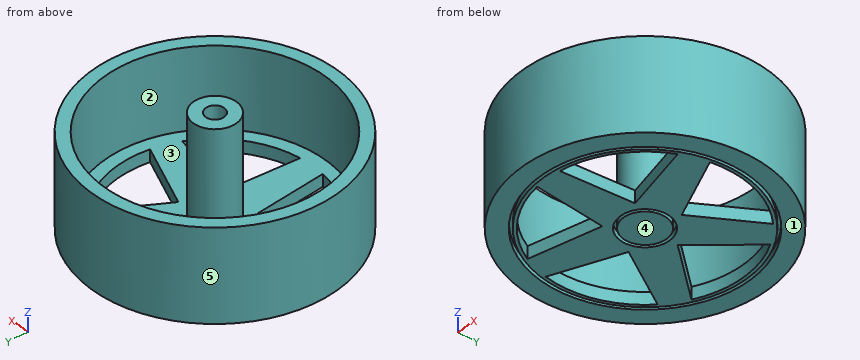
from build123d import *

# Parameters (mm, degrees)
F0_R      = 20
F1_DEPTH  = 15
F2_R      = 18
F3_DEPTH  = 13
F4_R      = 3.5
F4_R_2    = 1.5
F6_DEPTH  = 16
F7_DEPTH  = 2
F5_R      = 16.5
F5_R_2    = 17
F8_DEPTH  = 1
F9_R      = 4
F9_R_2    = 3.5
F10_DEPTH = 1


with BuildPart() as f1:
    # F0 (on Top) → F1 (new body)
    with BuildSketch(Plane.XY):
        Circle(F0_R)
    extrude(amount=F1_DEPTH)

    # F2 (on face) → F3 (cut)
    with BuildSketch(Plane.XY.offset(15)):
        Circle(F2_R)
    extrude(amount=-F3_DEPTH, mode=Mode.SUBTRACT)

    # F4 (on face) → F6 (join)
    with BuildSketch(Plane.XY.offset(2)):
        Circle(F4_R)
        Circle(F4_R_2, mode=Mode.SUBTRACT)
    extrude(amount=F6_DEPTH)

    # F5 (on face) → F7 (cut)
    with BuildSketch(Plane(origin=(0, 0, 0), x_dir=(1, 0, 0), z_dir=(0, 0, -1))):
        with BuildLine():
            Line((0, -5.352867), (-7.560142, -14.101215))
            ThreePointArc((-7.560142, -14.101215), (0, -16), (7.560142, -14.101215))
            Line((7.560142, -14.101215), (0, -5.352867))
        make_face()
        with BuildLine():
            Line((-5.090879, -1.654127), (-15.747264, 2.832607))
            ThreePointArc((-15.747264, 2.832607), (-15.216904, -4.944272), (-11.07484, -11.547637))
            Line((-11.07484, -11.547637), (-5.090879, -1.654127))
        make_face()
        with BuildLine():
            Line((-3.146336, 4.330561), (-2.172203, 15.851862))
            ThreePointArc((-2.172203, 15.851862), (-9.404564, 12.944272), (-14.404769, 6.964382))
            Line((-14.404769, 6.964382), (-3.146336, 4.330561))
        make_face()
        with BuildLine():
            ThreePointArc((14.404769, 6.964382), (9.404564, 12.944272), (2.172203, 15.851862))
            Line((2.172203, 15.851862), (3.146336, 4.330561))
            Line((3.146336, 4.330561), (14.404769, 6.964382))
        make_face()
        with BuildLine():
            Line((5.090879, -1.654127), (11.07484, -11.547637))
            ThreePointArc((11.07484, -11.547637), (15.216904, -4.944272), (15.747264, 2.832607))
            Line((15.747264, 2.832607), (5.090879, -1.654127))
        make_face()
    extrude(amount=-F7_DEPTH, mode=Mode.SUBTRACT)

    # F5 (on face) → F8 (cut)
    with BuildSketch(Plane(origin=(0, 0, 0), x_dir=(1, 0, 0), z_dir=(0, 0, -1))):
        Circle(F5_R)
        with BuildLine():
            ThreePointArc((-11.07484, -11.547637), (-15.216904, -4.944272), (-15.747264, 2.832607))
            Line((-15.747264, 2.832607), (-5.090879, -1.654127))
            Line((-5.090879, -1.654127), (-11.07484, -11.547637))
        make_face(mode=Mode.SUBTRACT)
        with BuildLine():
            ThreePointArc((7.560142, -14.101215), (0, -16), (-7.560142, -14.101215))
            Line((-7.560142, -14.101215), (0, -5.352867))
            Line((0, -5.352867), (7.560142, -14.101215))
        make_face(mode=Mode.SUBTRACT)
        with BuildLine():
            ThreePointArc((15.747264, 2.832607), (15.216904, -4.944272), (11.07484, -11.547637))
            Line((11.07484, -11.547637), (5.090879, -1.654127))
            Line((5.090879, -1.654127), (15.747264, 2.832607))
        make_face(mode=Mode.SUBTRACT)
        with BuildLine():
            ThreePointArc((-14.404769, 6.964382), (-9.404564, 12.944272), (-2.172203, 15.851862))
            Line((-2.172203, 15.851862), (-3.146336, 4.330561))
            Line((-3.146336, 4.330561), (-14.404769, 6.964382))
        make_face(mode=Mode.SUBTRACT)
        with BuildLine():
            Line((3.146336, 4.330561), (2.172203, 15.851862))
            ThreePointArc((2.172203, 15.851862), (9.404564, 12.944272), (14.404769, 6.964382))
            Line((14.404769, 6.964382), (3.146336, 4.330561))
        make_face(mode=Mode.SUBTRACT)
        Circle(F5_R_2)
        Circle(F5_R, mode=Mode.SUBTRACT)
    extrude(amount=-F8_DEPTH, mode=Mode.SUBTRACT)

    # F9 (on face) → F10 (cut)
    with BuildSketch(Plane(origin=(0, 0, 0), x_dir=(1, 0, 0), z_dir=(0, 0, -1))):
        Circle(F9_R)
        Circle(F9_R_2, mode=Mode.SUBTRACT)
    extrude(amount=-F10_DEPTH, mode=Mode.SUBTRACT)


solid = f1.part
Could you check a few things on this model? Use its own coordinates, in mm. Face numbers are marked on the shaded views. A direction names the side the tool comes from. Round coordinates to 2 decimals unless told otherwise and drop trailing zeros. Order: outer loops, then holes, each group sorted by start corner. A loop starts at its lowest first (then second) coordinate and runs counter-clockwise, first axis right, second up.
(1) Imagine slicing it at A-A (z = 2.5). Write out the boundary of the cut face in (x, y), plus the area to 3 significant figures.
Response values:
outline: circle Ø40 at (0, 0); circle Ø7 at (0, 0); hole circle Ø36 at (0, 0); hole circle Ø3 at (0, 0)
area: 270 mm2
(2) Which directions (+Z, -Z, +X, -X, +Y, -Y) give clear straight access to the entire face, cutting with the end or side of a thin tool? Please do the marked faces 1 and 2.
Response values:
face 1: -Z, +X, -X, +Y, -Y
face 2: +Z
(3) Imagine slicing it at C-C (y = 13). Write out the boundary of the cut face in (x, z).
Response values:
outline: (-15.2, 0) - (-10.95, 0) - (-10.95, 1) - (-10.16, 1) - (-10.16, 0) - (-6.61, 0) - (-6.61, 2) - (-12.45, 2) - (-12.45, 15) - (-15.2, 15) - close; (6.61, 0) - (10.16, 0) - (10.16, 1) - (10.95, 1) - (10.95, 0) - (15.2, 0) - (15.2, 15) - (12.45, 15) - (12.45, 2) - (6.61, 2) - close
(4) Imagine slicing it at B-B (y = -11). Write out the boundary of the cut face in (x, z).
Response values:
outline: (-16.7, 0) - (-12.96, 0) - (-12.96, 1) - (-12.3, 1) - (-12.3, 0) - (-11.62, 0) - (-11.62, 2) - (-14.25, 2) - (-14.25, 15) - (-16.7, 15) - close; (-2.58, 0) - (2.58, 0) - (2.58, 2) - (-2.58, 2) - close; (11.62, 0) - (12.3, 0) - (12.3, 1) - (12.96, 1) - (12.96, 0) - (16.7, 0) - (16.7, 15) - (14.25, 15) - (14.25, 2) - (11.62, 2) - close
(5) I'm going to push flat-ended pins straight in: pin 1 (1.5 mm diameter, centred on x = -1.5, z = 14.5, fed in from -Y); pin 2 (4 mm diameter, centred on y = 5.5, z = 2, fed in from +X); pin 3 (4 mm diameter, centred on x = 0.5, y = 15, fed in from +Z). Where does each tip first touch, or does it pass through?
Response values:
pin 1: stops at y = -19.99
pin 2: stops at x = 19.69
pin 3: stops at z = 2
(6) Please list where these lines run through material, in increasing order: line 1 along Y through (x, z) = (0, 7.5); line 2 along X through (y, z) = (-0.5, 11.5); line 3 along Z through (x, y) = (-1, 3.5).
Response values:
line 1: y = -20 to -18, -3.5 to -1.5, 1.5 to 3.5, 18 to 20
line 2: x = -19.99 to -17.99, -3.46 to -1.41, 1.41 to 3.46, 17.99 to 19.99
line 3: z = 1 to 2
(7) Imagine slicing it at D-D (y = 8.5). Write out the boundary of the cut face in (x, z).
Response values:
outline: (-18.1, 0) - (-14.72, 0) - (-14.72, 1) - (-14.14, 1) - (-14.14, 0) - (-13.56, 0) - (-13.56, 2) - (-15.87, 2) - (-15.87, 15) - (-18.1, 15) - close; (-9.23, 0) - (-2.72, 0) - (-2.72, 2) - (-9.23, 2) - close; (2.72, 0) - (9.23, 0) - (9.23, 2) - (2.72, 2) - close; (13.56, 0) - (14.14, 0) - (14.14, 1) - (14.72, 1) - (14.72, 0) - (18.1, 0) - (18.1, 15) - (15.87, 15) - (15.87, 2) - (13.56, 2) - close
(8) If we mould it in two halves opening along Y, with no side actions, what happens to the marked faces 3, 4 and 5? For each: released by +Y, released by -Y, zero draft, split by the parting line, or undercut.
Response values:
face 3: undercut
face 4: zero draft
face 5: split by the parting line
